Can you work these out from the drawing? Everything is in mm from the part's minimum corner. A direction names the side the tool comes from. Round coordinates to 2 decimals unless told otherwise and drop trailing zeros. Loops run counter-clockwise (first coordinate to the right, second up) from the corner with the lowest first, then second, coordinate; pieces in that order, holes last. Notation, with made-up numbers: M 39,49 L 81,49 A10 cw 81,64 Z; hole C -29,4.5 d2. An arc over 180 degrees is marked long. Answer in a Markdown table with one row per item.
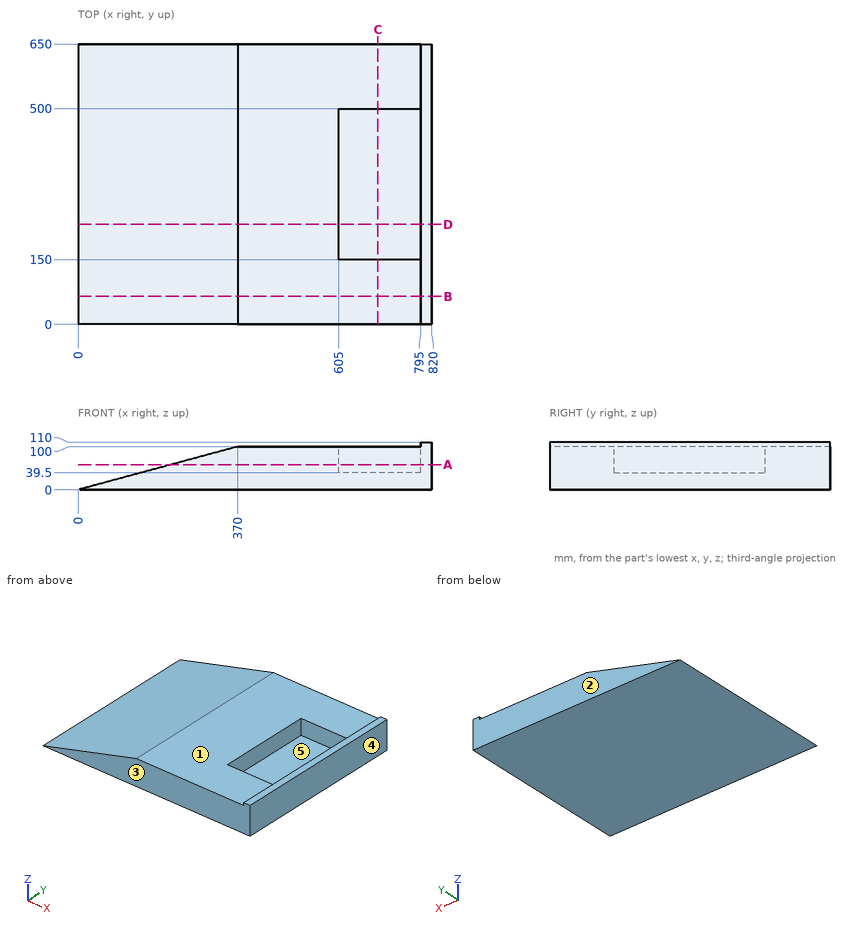
1) If we mould it in two halves opening along Y, with no side actions, what happens to the marked faces 3, 4 and 5? For each: released by +Y, released by -Y, zero draft, split by the parting line, or undercut.
Computed:
| item | result |
|---|---|
| face 3 | released by -Y |
| face 4 | zero draft |
| face 5 | undercut |
2) I want a section at C-C, the plane x = 695. Please give me the cut outline in (y, z), plus the area to 3 significant figures.
Computed:
| item | result |
|---|---|
| outline | M 0,0 L 650,0 L 650,100 L 500,100 L 500,39.5 L 150,39.5 L 150,100 L 0,100 Z |
| area | 43,800 mm² |
3) I want a section at D-D, the plane y = 232. Please give me the cut outline in (x, z), plus the area to 3 significant figures.
Computed:
| item | result |
|---|---|
| outline | M 0,0 L 820,0 L 820,110 L 795,110 L 795,39.5 L 605,39.5 L 605,100 L 370,100 Z |
| area | 52,300 mm² |
4) I want a section at A-A, the plane z = 58.5. Please give me the cut outline in (x, y), plus the area to 3 significant figures.
Computed:
| item | result |
|---|---|
| outline | M 216.45,0 L 820,0 L 820,650 L 216.45,650 Z; hole M 605,150 L 795,150 L 795,500 L 605,500 Z |
| area | 326,000 mm² |
5) I need wall thicknesses on line 1 (Y direction, x = 614, z = 69.5); line 2 (Z direction, x = 379.5, y = 70); line 3 (Z direction, x = 787.5, y = 321). Which ranges of each line are inside material? Lowest first, please.
Computed:
| item | result |
|---|---|
| line 1 | y = 0 to 150, 500 to 650 |
| line 2 | z = 0 to 100 |
| line 3 | z = 0 to 39.5 |
6) Which directions (+Z, -Z, +X, -X, +Y, -Y) give clear straight access to the entire face, cutting with the end or side of a thin tool? Please do the marked faces 1 and 2.
Computed:
| item | result |
|---|---|
| face 1 | +Z, -X, +Y, -Y |
| face 2 | +Z, -Z, +X, -X, +Y |
7) I want a section at B-B, the plane y = 65. Please give me the cut outline in (x, z).
Computed:
| item | result |
|---|---|
| outline | M 0,0 L 820,0 L 820,110 L 795,110 L 795,100 L 370,100 Z |
